Input: part model. Units: mm. Frame: model coordinates. A direction names the side the tool comes from. Round coordinates to 2 decimals unless told otherwise and drop trailing zeros. Order: outer loops, then holes, each group sorted by start corner. A loop starts at its lowest first (then second) coordinate and runs counter-clockwise, first axis right, second up. Notation, with made-up numbers: (-6, 29) -> (11, 29) arc R29 cw to (11, 54) -> close; hole circle Ø5 at (70, -9.5). An arc over 180 degrees is marked (long way). Use a Markdown table: item, result.
Autodesk Fusion 360 part; units mm, degrees
sketch "Sketch1" plane through (0, 0, 0) normal (0, 0, 1) x (1, 0, 0)
  line L0 (0, 0) -> (24, 0)
  line L1 (24, 0) -> (24, 19)
  line L2 (24, 19) -> (0, 19)
  line L3 (0, 19) -> (0, 0)
  dimension "d1" = 24
  dimension "d2" = 19
extrude "Extrude1" add sketch "Sketch1" along normal blind 2
sketch "Sketch4" plane through (0, 0, 2) normal (0, 0, 1) x (1, 0, 0)
  line L0 (0, 19) -> (0, 0)
  line L1 (0, 0) -> (24, 0)
  line L2 (24, 0) -> (24, 19)
  line L3 (24, 19) -> (0, 19)
  line L4 (24.6466, 21) -> (-2, 21)
  line L5 (-2, 21) -> (-2, -2)
  line L6 (-2, -2) -> (24.6466, -2)
  line L7 (24.6466, -2) -> (30, -2)
  line L8 (24.6466, 21) -> (30, 21)
  line L9 (30, 21) -> (30, -2) construction
  arc A0 (30, -2) -> (30, 21) centre (30, 9.5) ccw
  line L10 (24, 19) -> (30, 19)
  line L11 (24, 0) -> (30, 0)
  arc A1 (30, 0) -> (30, 19) centre (30, 9.5) ccw
  dimension "d23" = 2
  dimension "d24" = 2
  dimension "d25" = 2
  dimension "d26" = 6
  dimension "d27" = 19
extrude "Extrude5" add sketch "Sketch4" against normal blind 10
sketch "Sketch5" plane through (-2, 0, 0) normal (-1, 0, 0) x (0, 0, 1)
  line L0 (2, -2) -> (2, 21)
  line L1 (2, 21) -> (-8, 21)
  line L2 (-8, 21) -> (-8, -2)
  line L3 (-8, -2) -> (2, -2)
  line L4 (-8, 16.5) -> (0, 16.5)
  line L5 (0, 16.5) -> (0, 2.5)
  line L6 (0, 2.5) -> (-8, 2.5)
  line L7 (-8, 2.5) -> (-8, 16.5)
  dimension "d30" = 8
  dimension "d31" = 14
extrude "Extrude6" cut sketch "Sketch5" against normal up to surface (2 mm away) contours L2 L4 L5 L6 L7
fillet "Fillet1" radius 2 2 edges at (-2, 21, -3) (-2, -2, -3)
extrude "Extrude7" add 1 faces at (24, 6.3333, 0.6667) along direction (1, 0, 0) up to surface end surface at (33.2492, 18.4271, -4.6667)
sketch "Sketch6" plane through (0, 0, 0) normal (0, 0, -1) x (-1, 0, 0)
  line L0 (0, 16.5) -> (0, 19) construction
  line L1 (0, 19) -> (-30, 19)
  arc A0 (-30, 19) -> (-30, 0) centre (-30, 9.5) ccw
  line L2 (-30, 0) -> (0, 0)
  line L3 (0, 0) -> (0, 2.5) construction
  line L4 (0, 2.5) -> (2, 2.5) construction
  line L5 (2, 2.5) -> (2, 16.5) construction
  line L6 (2, 16.5) -> (0, 16.5) construction
  line L7 (-24, 19) -> (0, 19) construction
  line L8 (0, 19) -> (0, 0) construction
  line L9 (0, 0) -> (-24, 0) construction
  line L10 (-24, 0) -> (-24, 19) construction
  line L11 (-20.9, 16.5) -> (-3.1, 16.5) construction
  line L12 (-3.1, 16.5) -> (-3.1, 2.5) construction
  line L13 (-3.1, 2.5) -> (-20.9, 2.5) construction
  line L14 (-20.9, 2.5) -> (-20.9, 16.5) construction
  line L15 (-20.9, 2.5) -> (-3.1, 16.5) construction
  line L16 (-24, 19) -> (0, 0) construction
  circle A1 centre (-20.9, 16.5) radius 1
  circle A2 centre (-3.1, 16.5) radius 1
  circle A3 centre (-3.1, 2.5) radius 1
  circle A4 centre (-20.9, 2.5) radius 1
  point P0 (-24, 19)
  dimension "d38" = 17.8
  dimension "d39" = 14
  dimension "d40" = 2
extrude "Extrude8" cut sketch "Sketch6" against normal up to surface (2 mm away)
sketch "Sketch7" plane through (0, 0, 0) normal (0, 0, -1) x (-1, 0, 0)
  circle A0 centre (-3.1, 16.5) radius 1
  circle A1 centre (-20.9, 16.5) radius 1
  circle A2 centre (-3.1, 2.5) radius 1
  circle A3 centre (-20.9, 2.5) radius 1
  line L0 (0, 16.5) -> (0, 19)
  line L1 (0, 19) -> (-30, 19)
  arc A4 (-30, 19) -> (-30, 0) centre (-30, 9.5) ccw
  line L2 (-30, 0) -> (0, 0)
  line L3 (0, 0) -> (0, 2.5)
  line L4 (0, 2.5) -> (2, 2.5)
  line L5 (2, 2.5) -> (2, 16.5)
  line L6 (2, 16.5) -> (0, 16.5)
  circle A5 centre (-20.9, 16.5) radius 2
  circle A6 centre (-3.1, 16.5) radius 2
  circle A7 centre (-3.1, 2.5) radius 2
  circle A8 centre (-20.9, 2.5) radius 2
  dimension "d43" = 4
extrude "Extrude9" add sketch "Sketch7" along normal up to surface (6.4 mm away) contours A5 | A6 | A7 | A8
equation "d27 = 23 mm - 4 mm"
1) Cut plane D-D on x = 27.5. Return loops of the section in (y, z), and give its area (3 significant figures).
Answer key:
| item | result |
|---|---|
| outline | (-2, -8) -> (0, -8) -> (0, 2) -> (-2, 2) -> close; (0.33, 0) -> (18.67, 0) -> (18.67, 2) -> (0.33, 2) -> close; (19, -8) -> (21, -8) -> (21, 2) -> (19, 2) -> close |
| area | 76.7 mm^2 |
2) Ray query, probe 1 along Y at (x, z) = (20.9, -4); probe 2 along Y at (x, z) = (30, -7.5); probe 3 along Y at (x, z) = (4, -3.5). Return the intervals inside material, ascending.
Answer key:
| item | result |
|---|---|
| probe 1 | y = -2 to 0, 0.5 to 1.5, 3.5 to 4.5, 14.5 to 15.5, 17.5 to 18.5, 19 to 21 |
| probe 2 | y = -2 to 0, 19 to 21 |
| probe 3 | y = -2 to 0, 0.71 to 2.06, 2.94 to 4.29, 14.71 to 16.06, 16.94 to 18.29, 19 to 21 |
3) Contact query for flat-ended pins moving along their axis: P1, Ø3, axis at x = 20.5, y = 17, coming from the -Z side; P2, Ø0.6, axis at y = 0.5, z = 1, coming from the +X side; P3, Ø1, axis at y = 18, z = 1, coming from the +X side. Output: stop coordinate, or through.
Answer key:
| item | result |
|---|---|
| P1 | stops at z = -6.4 |
| P2 | stops at x = 37.52 |
| P3 | stops at x = 38.26 |
4) Set-up query: faces 1 (the face through (-1, 2.5, -4)), 2 (the face through (3.317, 17.476, -2.141)), 3 (the face through (39.498, 9.291, -3.944)). Return all of +Z, -Z, +X, -X, +Y, -Y with unobstructed straight access to the full face (end or side cutting, diameter ignored); none if empty.
Answer key:
| item | result |
|---|---|
| face 1 | -Z, -X |
| face 2 | +Z, -Z |
| face 3 | -Z |
5) Cut plane C-C on y = 9.5. Return loops of the section in (x, z), and give its area (3 significant figures).
Answer key:
| item | result |
|---|---|
| outline | (-2, 0) -> (39.5, 0) -> (39.5, -8) -> (41.5, -8) -> (41.5, 2) -> (-2, 2) -> close |
| area | 103 mm^2 |
6) Cut plane A-A on z = -0.75. State how many separate pieces and enclosed holes the cut face has, and give its area (3 significant figures).
Answer key:
| item | result |
|---|---|
| separate pieces | 5 |
| enclosed holes | 4 |
| area | 240 mm^2 |
7) Draft query along Y for faces 4 (the face through (41.497, 9.247, -2.93)), 5 (the face through (15, -2, -3)), 6 (the face through (-1, 16.5, -4)). Return one class per face: released by +Y, released by -Y, zero draft, split by the parting line, or undercut.
Answer key:
| item | result |
|---|---|
| face 4 | split by the parting line |
| face 5 | released by -Y |
| face 6 | undercut |
8) Cut plane B-B on x = 20.9. Return loops of the section in (y, z), and give its area (3 significant figures).
Answer key:
| item | result |
|---|---|
| outline | (-2, -8) -> (0, -8) -> (0, 0) -> (0.5, 0) -> (0.5, -6.4) -> (1.5, -6.4) -> (1.5, 2) -> (-2, 2) -> close; (3.5, -6.4) -> (4.5, -6.4) -> (4.5, 0) -> (14.5, 0) -> (14.5, -6.4) -> (15.5, -6.4) -> (15.5, 2) -> (3.5, 2) -> close; (17.5, -6.4) -> (18.5, -6.4) -> (18.5, 0) -> (19, 0) -> (19, -8) -> (21, -8) -> (21, 2) -> (17.5, 2) -> close |
| area | 95.6 mm^2 |
